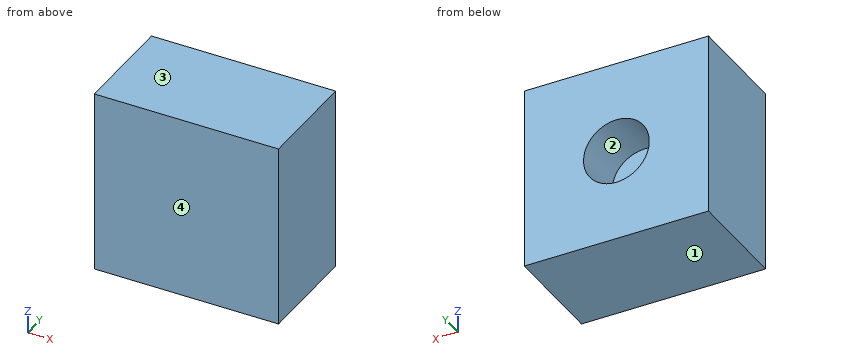
Autodesk Inventor part; units mm, degrees
ref_plane "YZ Plane" through (0, 0, 0) normal (1, 0, 0) x (0, 1, 0)
ref_plane "XZ Plane" through (0, 0, 0) normal (0, 1, 0) x (-1, 0, 0)
ref_plane "XY Plane" through (0, 0, 0) normal (0, 0, 1) x (1, 0, 0)
sketch "Boceto1" plane through (0, 0, 0) normal (0, 1, 0) x (-1, 0, 0)
  line L0 (0, 0) -> (-1400, 0)
  line L1 (-1400, 0) -> (-1400, -1400)
  line L2 (-1400, -1400) -> (0, -1400)
  line L3 (0, -1400) -> (0, 0)
  dimension "d0" = 1400
  dimension "d1" = 1400
extrude "Extrusión1" add sketch "Boceto1" along normal blind 800
sketch "Boceto2" plane through (0, 800, 0) normal (0, 1, 0) x (1, 0, 0)
  line L0 (0, 0) -> (800, 0)
  circle A0 centre (700, 700) radius 250
  line L1 (0, 1400) -> (0, 0)
  line L2 (1400, 1400) -> (0, 1400)
  dimension "d6" = 500
  dimension "d9" = 700
  dimension "d10" = 700
extrude "Extrusión2" cut sketch "Boceto2" against normal blind 400
properties part number "Soporte"
Geometry: final body of the model. Coordinates: model frame, mm. Face numbers are marked on the shaded views. Round coordinates to 2 decimals unless told otherwise and drop trailing zeros. Order: outer loops, then holes, each group sorted by start corner. A loop starts at its lowest first (then second) coordinate and runs counter-clockwise, first axis right, second up. Notation, with made-up numbers: (-28, -9.75) - (5, -9.75) arc R17 ccw to (5, 9.25) - close; hole circle Ø6 at (2.5, -6). An arc over 180 degrees is marked (long way). Write item = value, one per line. Start each with the question number.
Q1. Pin query (flat end, axial travel): pin 1 (5 mm diameter, centred on y = 309, z = -194.5, fed in from -X). Return the tip coordinate at first contact, or that it passes through.
Q2. Cut plane C-C on z = -700. Return the cut outline in (x, y).
Q3. Cut plane B-B on x = 700. Return the cut outline in (y, z), and give its area (3 significant figures).
Q4. Ray query, line 1 (X direction, y = 640.5, z = -700); line 2 (Z direction, x = 700, y = 503); line 3 (X direction, y = 687, z = -687). Return the intervals inside material, ascending. Write a range as from..to.
Q5. Pull-direction query (Z, two-part tool) for the marked faces 1, 2, 3 and 4; classes: +Z half, -Z half, draft (parallel to the pull), parting line (faces both ways), or undercut.
Q6. Cut plane A-A on y = 429.5. Return the cut outline in (x, z), and give its area (3 significant figures).
Outcome:
q1.pin_1 = 0
q2.outline = (0, 0) - (1400, 0) - (1400, 800) - (950, 800) - (950, 400) - (450, 400) - (450, 800) - (0, 800) - close
q3.outline = (0, -1400) - (800, -1400) - (800, -950) - (400, -950) - (400, -450) - (800, -450) - (800, 0) - (0, 0) - close
q3.area = 920,000 mm^2
q4.line_1 = 0..450, 950..1400
q4.line_2 = -1400..-950, -450..0
q4.line_3 = 0..450.34, 949.66..1400
q5.face_1 = -Z half
q5.face_2 = undercut
q5.face_3 = +Z half
q5.face_4 = draft
q6.outline = (0, -1400) - (1400, -1400) - (1400, 0) - (0, 0) - close; hole circle Ø500 at (700, -700)
q6.area = 1,760,000 mm^2
